from build123d import *

# Parameters (mm, degrees)
SKETCH1_R           = 0.5
SKETCH1_W           = 1.5
SKETCH1_H           = 0.5
BOSS_EXTRUDE1_DEPTH = 0.3
SKETCH2_R           = 0.15
CUT_EXTRUDE1_DEPTH  = 0.3
CIRPATTERN1_COUNT   = 4
SKETCH5_R           = 0.25
CUT_EXTRUDE3_DEPTH  = 0.3


with BuildPart() as part:
    # Sketch1 → Boss-Extrude1 (new body)
    with BuildSketch(Plane(origin=(0, 0, 0), x_dir=(1, 0, 0), z_dir=(0, 1, 0))):
        with BuildLine():
            Line((0, 0), (2.5, 0))
            Line((2.5, 0), (2.5, 6.5))
            ThreePointArc((2.5, 6.5), (1.25, 7.75), (0, 6.5))
            Line((0, 6.5), (0, 0))
        make_face()
        with Locations(Location((1.25, 6.5, 0), (0, 0, 270))):
            Circle(SKETCH1_R, mode=Mode.SUBTRACT)
        with Locations((1.25, 0.75)):
            Rectangle(SKETCH1_W, SKETCH1_H, mode=Mode.SUBTRACT)
    extrude(amount=BOSS_EXTRUDE1_DEPTH)

    # Sketch2 → Cut-Extrude1 (cut)
    with BuildSketch(Plane(origin=(0, 0.3, 0), x_dir=(1, 0, 0), z_dir=(0, 1, 0))):
        with Locations(Location((0.25, 6.5, 0), (0, 0, 270))):
            Circle(SKETCH2_R)
    cut_extrude1 = extrude(amount=-CUT_EXTRUDE1_DEPTH, mode=Mode.SUBTRACT)

    # CirPattern1: Cut-Extrude1 ×4 about axis
    cirpattern1_axis = Axis((1.25, 0, -6.5), (0, 1, 0))
    for i in range(1, CIRPATTERN1_COUNT):
        add(cut_extrude1.rotate(cirpattern1_axis, i * 360 / CIRPATTERN1_COUNT), mode=Mode.SUBTRACT)

    # Sketch5 → Cut-Extrude3 (cut)
    with BuildSketch(Plane(origin=(0, 0.3, 0), x_dir=(1, 0, 0), z_dir=(0, 1, 0))):
        with Locations(Location((1.25, 3.25, 0), (0, 0, 270))):
            Circle(SKETCH5_R)
    extrude(amount=-CUT_EXTRUDE3_DEPTH, mode=Mode.SUBTRACT)


solid = part.part
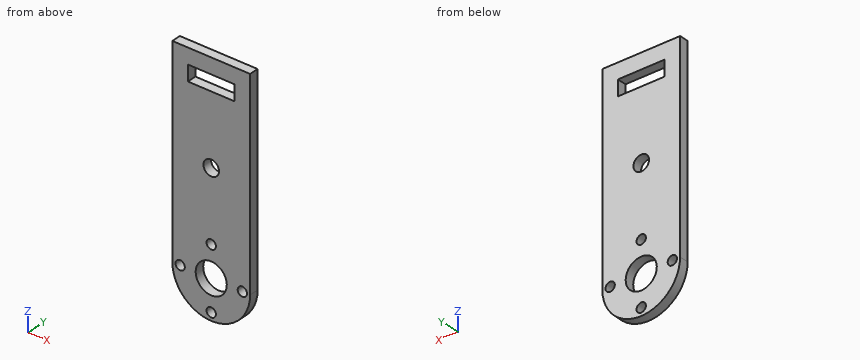
The model under review builds one solid part; all positions refer to its coordinate system, in mm. Round coordinates to 2 decimals unless told otherwise and drop trailing zeros. Order: outer loops, then holes, each group sorted by start corner. A loop starts at its lowest first (then second) coordinate and runs counter-clockwise, first axis right, second up. Notation, with made-up numbers: (83.5, 40.5) - (130.5, 40.5) arc R19 ccw to (130.5, 50.5) - close; hole circle Ø3 at (47, 19.5). An arc over 180 degrees is marked (long way). Use one line per item in the form item = value.
Q1. Add section C-C on y = 0.25. Give the boundary of the cut face in (x, z), then the cut area to 3 significant figures.
Response values:
outline = (0, -6.5) arc R1.25 ccw to (2.5, -6.5) - (2.5, 0) - (0, 0) - close; hole circle Ø0.3 at (0.25, -6.5); hole (0.5, -1) - (2, -1) - (2, -0.5) - (0.5, -0.5) - close; hole circle Ø1 at (1.25, -6.5); hole circle Ø0.5 at (1.25, -3.25); hole circle Ø0.3 at (1.25, -7.5); hole circle Ø0.3 at (1.25, -5.5); hole circle Ø0.3 at (2.25, -6.5)
area = 16.7 mm^2
Q2. To check wall thickness, follow line 1 (X direction, y = 0.2, z = -7.5); line 2 (X direction, y = 0.1, z = -3.25); line 3 (Z direction, x = 0.2, y = 0.1). State the ranges of each line that lie inside material, in increasing order.
Response values:
line_1 = 0.5 to 1.1, 1.4 to 2
line_2 = 0 to 1, 1.5 to 2.5
line_3 = -7.18 to -6.64, -6.36 to 0
Q3. Clearance check with a flat-ended pin moving along its axis: P1, Ø1, axis at x = 0.5, z = -6.5, coming from the -Y side. State where the tip first meets the part, or that it passes through.
Response values:
P1 = 0
Q4. Add section D-D on x = 1.85. Give the boundary of the cut face in (y, z), then the cut area to 3 significant figures.
Response values:
outline = (0, -7.6) - (0.3, -7.6) - (0.3, -1) - (0, -1) - close; (0, -0.5) - (0.3, -0.5) - (0.3, 0) - (0, 0) - close
area = 2.13 mm^2
Q5. Add section A-A on x = 1.25. Give the boundary of the cut face in (y, z), then the cut area to 4 significant figures.
Response values:
outline = (0, -7.75) - (0.3, -7.75) - (0.3, -7.65) - (0, -7.65) - close; (0, -7.35) - (0.3, -7.35) - (0.3, -7) - (0, -7) - close; (0, -6) - (0.3, -6) - (0.3, -5.65) - (0, -5.65) - close; (0, -5.35) - (0.3, -5.35) - (0.3, -3.5) - (0, -3.5) - close; (0, -3) - (0.3, -3) - (0.3, -1) - (0, -1) - close; (0, -0.5) - (0.3, -0.5) - (0.3, 0) - (0, 0) - close
area = 1.545 mm^2
Q6. Add section B-B on z = -7.5. Give the boundary of the cut face in (x, y).
Response values:
outline = (0.5, 0) - (1.1, 0) - (1.1, 0.3) - (0.5, 0.3) - close; (1.4, 0) - (2, 0) - (2, 0.3) - (1.4, 0.3) - close
